The listing builds one solid part. Answer for the finished solid, in the listing's coordinates (mm). Face numbers are marked on the shaded views. A direction names the side the tool comes from. Coordinates: 2 decimals unless noted, no trailing zeros. Write each loop counter-clockwise with the first axis right and the second up, starting at its lowest first coordinate (ties: lowest second). Pieces come first, ordered by that corner, then holes.
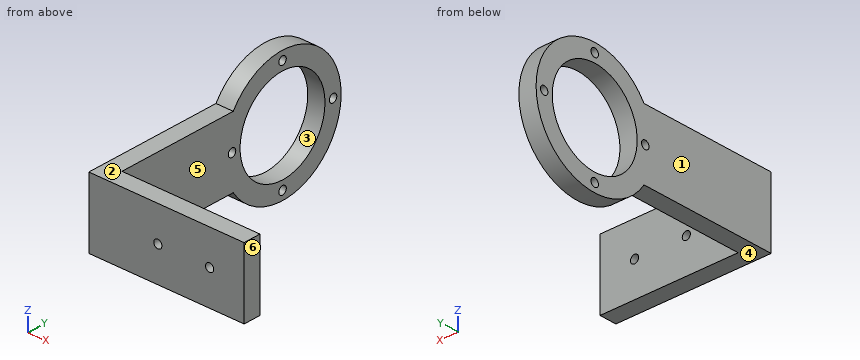
Autodesk Inventor part; units mm, degrees
ref_plane "YZ Plane" through (0, 0, 0) normal (1, 0, 0) x (0, 1, 0)
ref_plane "XZ Plane" through (0, 0, 0) normal (0, 1, 0) x (-1, 0, 0)
ref_plane "XY Plane" through (0, 0, 0) normal (0, 0, 1) x (1, 0, 0)
sketch "Sketch1" plane through (0, 0, 0) normal (1, 0, 0) x (0, 1, 0)
  circle A0 centre (0, 0) radius 17.018
  circle A1 centre (0, 0) radius 23.495
  line L0 (-19.7668, 12.7) -> (-70.7247, 12.7)
  line L1 (-70.7247, 12.7) -> (-70.7247, -12.7)
  line L2 (-70.7247, -12.7) -> (-19.7668, -12.7)
  dimension "d0" = 6.477
  dimension "d1" = 34.036
  dimension "d7" = 25.4
extrude "Extrusion1" add sketch "Sketch1" along normal blind 6.35
sketch "Sketch2" plane through (6.35, 0, 0) normal (1, 0, 0) x (0, 0, -1)
  line L0 (-12.7, -19.7668) -> (-12.7, -70.7247)
  line L1 (12.7, -70.7247) -> (12.7, -19.7668)
  line L2 (-12.7, -70.7247) -> (12.7, -70.7247)
  line L3 (12.7, -70.7247) -> (12.7, -64.3747)
  line L4 (12.7, -64.3747) -> (-12.7, -64.3747)
  line L5 (-12.7, -64.3747) -> (-12.7, -70.7247)
  point P0 (0, 0)
  dimension "d10" = 6.35
extrude "Extrusion2" add sketch "Sketch2" along normal blind 50.8
sketch "Sketch3" plane through (0, -70.7247, -12.7) normal (0, -1, 0) x (1, 0, 0)
  circle A0 centre (25.4, 12.7) radius 1.5
  circle A1 centre (44.45, 12.7) radius 1.5
  line L0 (0, 25.4) -> (57.15, 25.4)
  line L1 (57.15, 25.4) -> (57.15, 0)
  line L2 (0, 25.4) -> (0, 0)
  point P0 (0, 12.7)
  dimension "d14" = 12.7
  dimension "d15" = 12.7
  dimension "d16" = 3
  dimension "d17" = 3
  dimension "d18" = 12.7
  dimension "d19" = 25.4
extrude "Extrusion3" cut sketch "Sketch3" against normal blind 50.8
sketch "Sketch4" plane through (6.35, 0, 0) normal (1, 0, 0) x (0, 0, -1)
  line L0 (0, 23.4884) -> (0, 17.018)
  circle A0 centre (0, 0) radius 17.018
  circle A1 centre (0, 20.2532) radius 1.5
  circle A2 centre (-20.2532, 0) radius 1.5
  circle A3 centre (0, -20.2532) radius 1.5
  circle A4 centre (20.2532, 0) radius 1.5
  dimension "d22" = 3
  dimension "d25" = 360
extrude "Extrusion4" cut sketch "Sketch4" against normal blind 50.8 contours A1 L0 | L0 A1 | A2 | A3 | A4
properties part number "LED Hinge"
1. Section B-B on y = 0 is taken. Give the vertices of the cut face in (x, z) (3 decimals), then the cut area to 3 significant figures.
Results found:
outline: (0, -23.495) - (6.35, -23.495) - (6.35, -21.753) - (0, -21.753) - close; (0, -18.753) - (6.35, -18.753) - (6.35, -17.018) - (0, -17.018) - close; (0, 17.018) - (6.35, 17.018) - (6.35, 18.753) - (0, 18.753) - close; (0, 21.753) - (6.35, 21.753) - (6.35, 23.495) - (0, 23.495) - close
area: 44.2 mm2
2. A tool of negligible diameter and unlimited length cuts with its end or side. For the marked faces 4, 5 and 6, from which of +Z, -Z, +X, -X, +Y, -Y can it reach the whole face along a straight path? Write none if from no direction.
Results found:
face 4: -Z, +X, -X, -Y
face 5: +Z, -Z, +X, +Y
face 6: +Z, -Z, +X, +Y, -Y
3. Find the intervals of material crossed by L1, parallel to X at y = 13.5, z = 15.5; L2, parallel to Y at x = 34, z = -7.5; L3, parallel to Y at x = 2, z = 8.5, in increasing order.
Results found:
L1: x = 0 to 6.35
L2: y = -70.72 to -64.37
L3: y = -70.72 to -14.74, 14.74 to 21.9
4. Section C-C on x = 25.4 is taken. Give the vertices of the cut face in (y, z).
Results found:
outline: (-70.72, -12.7) - (-64.37, -12.7) - (-64.37, -1.5) - (-70.72, -1.5) - close; (-70.72, 1.5) - (-64.37, 1.5) - (-64.37, 12.7) - (-70.72, 12.7) - close
5. For a pull along Z with two mould halves and no side action, classify the marked faces 1, 2 and 3 as pulls with the +Z half, pulls with the -Z half, needs draft (parallel to the pull), parting line crosses it, or undercut.
Results found:
face 1: needs draft
face 2: pulls with the +Z half
face 3: undercut
6. Section A-A on z = 0 is taken. Give the vertices of the cut face in (x, y) (3 decimals).
Results found:
outline: (0, -70.725) - (23.9, -70.725) - (23.9, -64.375) - (6.35, -64.375) - (6.35, -21.753) - (0, -21.753) - close; (0, -18.753) - (6.35, -18.753) - (6.35, -17.018) - (0, -17.018) - close; (0, 17.018) - (6.35, 17.018) - (6.35, 18.753) - (0, 18.753) - close; (0, 21.753) - (6.35, 21.753) - (6.35, 23.495) - (0, 23.495) - close; (26.9, -70.725) - (42.95, -70.725) - (42.95, -64.375) - (26.9, -64.375) - close; (45.95, -70.725) - (57.15, -70.725) - (57.15, -64.375) - (45.95, -64.375) - close
7. Section D-D on z = -9 is taken. Give the vertices of the cut face in (x, y), then the cut area to 3 significant figures.
Results found:
outline: (0, -70.72) - (57.15, -70.72) - (57.15, -64.37) - (6.35, -64.37) - (6.35, -14.44) - (0, -14.44) - close; (0, 14.44) - (6.35, 14.44) - (6.35, 21.7) - (0, 21.7) - close
area: 726 mm2
8. Flat-ended cylindrical pins translate along their axes: P1, Ø1.5, axis at x = 41.5, z = 5.5, coming from the +Y side; P2, Ø3, axis at y = -27, z = -3, coming from the +X side. Find the tip coordinate at first contact, or state that the pin passes through.
Results found:
P1: stops at y = -64.37
P2: stops at x = 6.35
